Work out the finished part from the listing and answer in its coordinate system (mm). Face numbers are marked on the shaded views. A direction names the side the tool comes from. Give positions to 0.01 mm unless a question says otherwise; leave off trailing zeros. Write each loop counter-clockwise with the first axis right and the second up, starting at its lowest first coordinate (ties: lowest second). Pieces come first, ordered by that corner, then holes. Notation, with made-up numbers: (-18, 79) -> (38, 79) arc R18 cw to (38, 110) -> close; hole circle Ø10 at (79, 28.25). An arc over 180 degrees is marked (long way). Use a Markdown table: item, result. Add a question column.
Q1. Section B-B, the plane x = 25 is taken. Give the vertices of the cut face in (y, z).
Q2. Each of these flat-tipped pins is pushed along its axis until it touches: pin 1 Ø3 at (y, z) = (6, 19) entering from -X; pin 2 Ø6 at (x, y) = (63, 50.5) entering from -Z; pin 3 Ø1.5 at (x, z) = (96, 11.5) entering from -Y; pin 4 Ø4 at (y, z) = (129, 11.5) entering from +X. Where does it stop, or does it pass through?
Q3. Consider line 1 (Z direction, x = 54, y = 98.5); line 2 (X direction, y = 144.2, z = 10.5); line 3 (X direction, y = 51, z = 26.5). Determine where each line is inside the solid, lowest interval first.
Q4. Section A-A, the plane y = 79.5 is taken. Give the vertices of the cut face in (x, z).
Q5. Section C-C, the plane y = 40 is taken. Give the vertices of the cut face in (x, z), plus the area to 3 significant figures.
Q6. For the marked faces 1, 2 and 3, determine the directions among +Z, -Z, +X, -X, +Y, -Y from which every point of the face is accessible in a straight line to the end or side of a thin tool.
Q7. For a pull along X with two mould halves and no side action, classify the marked faces 4 and 5 as pulls with the +X half, pulls with the -X half, needs draft (parallel to the pull), parting line crosses it, or undercut.
Autodesk Inventor part; units mm, degrees
ref_plane "Work Plane1" through (0, 0, 12.5) normal (0, 0, -1) x (-1, 0, 0)
ref_plane "Work Plane2" through (0, 0, 27) normal (0, 0, 1) x (1, 0, 0)
ref_plane "YZ Plane" through (0, 0, 0) normal (1, 0, 0) x (0, 1, 0)
sketch "Sketch1" plane through (0, 0, 0) normal (0, 0, 1) x (1, 0, 0)
  line L0 (33.3378, 145.104) -> (83.3378, 145.104)
  line L1 (83.3378, 145.104) -> (83.3378, 5.104)
  line L2 (83.3378, 5.104) -> (33.3378, 5.104)
  line L3 (33.3378, 5.104) -> (33.3378, 145.104)
  line L4 (33.3378, 90.104) -> (33.3378, 60.104)
  line L5 (83.3378, 90.104) -> (83.3378, 60.104)
  point P0 (0, 0)
  dimension "d0" = 140
  dimension "d1" = 50
extrude "Extrusion1" add sketch "Sketch1" along normal blind 30
sketch "Sketch2" plane through (0, 0, 30) normal (0, 0, 1) x (1, 0, 0)
  line L0 (35.8378, 142.604) -> (80.8378, 142.604)
  line L1 (80.8378, 142.604) -> (80.8378, 7.604)
  line L2 (80.8378, 7.604) -> (35.8378, 7.604)
  line L3 (35.8378, 7.604) -> (35.8378, 142.604)
  line L4 (83.3378, 145.104) -> (33.3378, 145.104)
  line L5 (83.3378, 5.104) -> (83.3378, 145.104)
  line L6 (33.3378, 5.104) -> (83.3378, 5.104)
  line L7 (33.3378, 145.104) -> (33.3378, 5.104)
  point P0 (0, 0)
  point P1 (58.3378, 142.604)
  dimension "d4" = 2.5
  dimension "d5" = 2.5
  dimension "d6" = 2.5
  dimension "d7" = 2.5
extrude "Extrusion2" cut sketch "Sketch2" against normal blind 27 contours L0 L1 L2 L3
sketch "Sketch3" plane through (33.3378, 5.104, 0) normal (0, -1, 0) x (1, 0, 0)
  line L0 (7, 30) -> (37, 30)
  line L1 (37, 30) -> (37, 15)
  line L2 (37, 15) -> (7, 15)
  line L3 (7, 15) -> (7, 30)
  line L4 (0, 0) -> (50, 0)
  line L5 (0, 0) -> (0, 30)
  line L6 (0, 30) -> (50, 30)
  line L7 (10, 15) -> (35, 15)
  line L8 (35, 15) -> (35, 3)
  line L9 (35, 3) -> (10, 3)
  line L10 (10, 3) -> (10, 15)
  point P0 (-33.3378, 0)
  point P1 (37, 22.5)
  point P2 (10, 9)
  dimension "d10" = 15
  dimension "d11" = 30
  dimension "d12" = 7
  dimension "d13" = 0
  dimension "d14" = 25
  dimension "d15" = 10
  dimension "d16" = 3
extrude "Extrusion3" cut sketch "Sketch3" against normal blind 27
sketch "Sketch4" plane through (0, 0, 0) normal (0, 0, -1) x (-1, 0, 0)
  circle A0 centre (-74.8378, 13.604) radius 1.5
  circle A1 centre (-41.8378, 13.604) radius 1.5
  circle A2 centre (-41.8378, 99.604) radius 1.5
  circle A3 centre (-74.8378, 99.604) radius 1.5
  circle A4 centre (-41.8378, 111.604) radius 1.5
  circle A5 centre (-74.8378, 111.604) radius 1.5
  line L0 (-83.3378, 5.104) -> (-83.3378, 145.104)
  line L1 (-33.3378, 145.104) -> (-33.3378, 5.104)
  line L2 (-33.3378, 5.104) -> (-83.3378, 5.104)
  line L3 (-83.3378, 145.104) -> (-33.3378, 145.104)
  point P0 (0, 0)
  dimension "d19" = 8.5
  dimension "d20" = 8.5
  dimension "d21" = 8.5
  dimension "d22" = 8.5
  dimension "d23" = 3
  dimension "d24" = 3
  dimension "d25" = 8.5
  dimension "d26" = 8.5
  dimension "d27" = 8.5
  dimension "d28" = 8.5
  dimension "d29" = 3
  dimension "d30" = 3
  dimension "d31" = 3
  dimension "d32" = 3
  dimension "d33" = 12
  dimension "d34" = 12
  dimension "d35" = 33.5
  dimension "d36" = 33.5
extrude "Extrusion4" cut sketch "Sketch4" against normal blind 27 contours A0 | A1 | A2 | A3 | A4 | A5
sketch "Sketch5" plane through (33.3378, 145.104, 0) normal (0, 1, 0) x (1, 0, 0)
  circle A0 centre (35.5, -10.5) radius 2.5
  circle A1 centre (10.5, -10.5) radius 2.5
  line L0 (50, 0) -> (50, -30)
  line L1 (50, 0) -> (0, 0)
  point P0 (-33.3378, 0)
  dimension "d39" = 5
  dimension "d40" = 5
  dimension "d41" = 25
  dimension "d42" = 14.5
  dimension "d43" = 10.5
  dimension "d44" = 10.5
extrude "Extrusion5" cut sketch "Sketch5" against normal blind 27
sketch "Sketch6" plane through (33.3378, 5.104, 0) normal (0, -1, 0) x (1, 0, 0)
  point P0 (-33.3378, 0)
ref_plane "Work Plane1" through (0, 0, 12.5) normal (0, 0, -1) x (-1, 0, 0)
sketch "Sketch7" plane through (0, 0, 12.5) normal (0, 0, -1) x (-1, 0, 0)
  line L0 (-83.3378, 5.104) -> (-83.3378, 145.104)
  line L1 (-83.3378, 90.104) -> (-103.3378, 90.104)
  line L2 (-103.3378, 90.104) -> (-103.3378, 60.104)
  line L3 (-103.3378, 60.104) -> (-83.3378, 60.104)
  line L4 (-83.3378, 60.104) -> (-83.3378, 90.104)
  line L5 (-83.3378, 145.104) -> (-33.3378, 145.104)
  line L6 (-88.3378, 65.104) -> (-98.3378, 65.104)
  line L7 (-98.3378, 65.104) -> (-98.3378, 85.104)
  line L8 (-98.3378, 85.104) -> (-88.3378, 85.104)
  line L9 (-88.3378, 85.104) -> (-88.3378, 65.104)
  line L10 (-33.3378, 145.104) -> (-33.3378, 5.104)
  line L11 (-13.3378, 90.104) -> (-33.3378, 90.104)
  line L12 (-33.3378, 90.104) -> (-33.3378, 60.104)
  line L13 (-33.3378, 60.104) -> (-13.3378, 60.104)
  line L14 (-13.3378, 60.104) -> (-13.3378, 90.104)
  line L15 (-18.3378, 85.104) -> (-28.3378, 85.104)
  line L16 (-28.3378, 85.104) -> (-28.3378, 65.104)
  line L17 (-28.3378, 65.104) -> (-18.3378, 65.104)
  line L18 (-18.3378, 65.104) -> (-18.3378, 85.104)
  point P0 (0, 0)
  point P1 (-93.3378, 60.104)
  dimension "d56" = 20
  dimension "d57" = 30
  dimension "d58" = 55
  dimension "d59" = 5
  dimension "d60" = 20
  dimension "d61" = 30
  dimension "d62" = 55
  dimension "d63" = 5
extrude "Extrusion6" add sketch "Sketch7" along normal mid plane 5
ref_plane "Work Plane2" through (0, 0, 27) normal (0, 0, 1) x (1, 0, 0)
sketch "Sketch8" plane through (0, 0, 27) normal (0, 0, 1) x (1, 0, 0)
  line L0 (80.8378, 142.604) -> (80.8378, 7.604)
  line L1 (35.8378, 7.604) -> (35.8378, 142.604)
  line L2 (80.8378, 107.604) -> (35.8378, 107.604)
  line L3 (35.8378, 107.604) -> (35.8378, 82.604)
  line L4 (35.8378, 82.604) -> (80.8378, 82.604)
  line L5 (80.8378, 82.604) -> (80.8378, 107.604)
  line L6 (35.8378, 142.604) -> (80.8378, 142.604)
  point P0 (0, 0)
  dimension "d67" = 35
  dimension "d68" = 25
extrude "Extrusion7" add sketch "Sketch8" against normal blind 10 contours L0 L4 L1 L2
sketch "Sketch9" plane through (35.8378, 82.604, 27) normal (0, -1, 0) x (1, 0, 0)
  line L0 (43, -2) -> (2, -2)
  line L1 (2, -2) -> (2, -8)
  line L2 (2, -8) -> (43, -8)
  line L3 (43, -8) -> (43, -2)
  line L4 (4.5, -12) -> (4.5, 3)
  line L5 (0, 0) -> (45, 0)
  line L6 (45, -10) -> (0, -10)
  line L7 (0, -10) -> (0, 0)
  point P0 (-35.8378, -27)
  point P1 (45, 3)
  point P2 (4.5, -2)
  point P3 (4.5, -8)
  dimension "d72" = 2
  dimension "d73" = 2
  dimension "d74" = 2
  dimension "d75" = 2
extrude "Extrusion8" cut sketch "Sketch9" against normal blind 27 contours L3 L2 L4 L0
properties part number "arduino mould_3r"
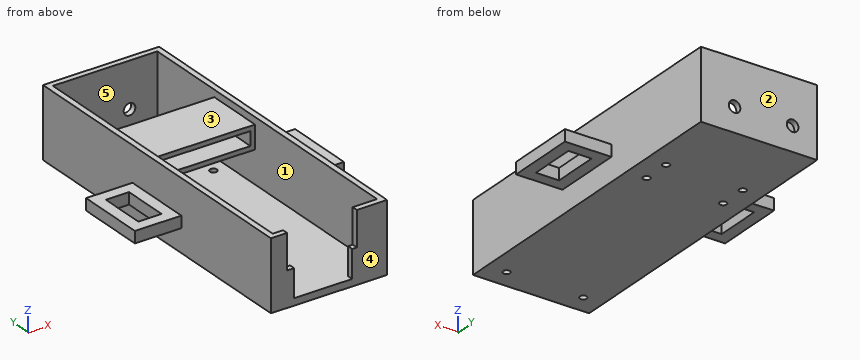
Result set:
| question | item | result |
|---|---|---|
| 1 | outline | (60.1, 10) -> (65.1, 10) -> (65.1, 15) -> (60.1, 15) -> close; (85.1, 10) -> (90.1, 10) -> (90.1, 15) -> (85.1, 15) -> close |
| 2 | pin 1 | stops at x = 33.34 |
| 2 | pin 2 | stops at z = 0 |
| 2 | pin 3 | stops at y = 60.1 |
| 2 | pin 4 | stops at x = 83.34 |
| 3 | line 1 | z = 0 to 3, 17 to 19, 25 to 27 |
| 3 | line 2 | x = 33.34 to 41.34, 46.34 to 66.34, 71.34 to 83.34 |
| 3 | line 3 | x = 33.34 to 35.84, 80.84 to 83.34 |
| 4 | outline | (13.34, 10) -> (18.34, 10) -> (18.34, 15) -> (13.34, 15) -> close; (28.34, 10) -> (33.34, 10) -> (33.34, 0) -> (83.34, 0) -> (83.34, 10) -> (88.34, 10) -> (88.34, 15) -> (83.34, 15) -> (83.34, 30) -> (80.84, 30) -> (80.84, 3) -> (35.84, 3) -> (35.84, 30) -> (33.34, 30) -> (33.34, 15) -> (28.34, 15) -> close; (98.34, 10) -> (103.34, 10) -> (103.34, 15) -> (98.34, 15) -> close |
| 5 | outline | (33.34, 0) -> (83.34, 0) -> (83.34, 30) -> (80.84, 30) -> (80.84, 3) -> (35.84, 3) -> (35.84, 30) -> (33.34, 30) -> close |
| 5 | area | 285 mm2 |
| 6 | face 1 | none |
| 6 | face 2 | +Z, -Z, +X, -X, +Y |
| 6 | face 3 | +Z |
| 7 | face 4 | needs draft |
| 7 | face 5 | undercut |
